```python
from build123d import *

# Parameters (mm, degrees)
ESBO_O1_W                = 140
ESBO_O1_H                = 100
RESSALTO_EXTRUS_O1_DEPTH = 1.5
RESSALTO_EXTRUS_O2_DEPTH = 3
ESBO_O2_R                = 1.5
CORTE_EXTRUS_O1_DEPTH    = 95.451045521
CUT_EXTRUDE1_DEPTH       = 95.451045521
CUT_EXTRUDE1_DEPTH_BACK  = 95.451045521
SKETCH1_R                = 1.7
CUT_EXTRUDE4_DEPTH       = 95.415305963
CUT_EXTRUDE4_DEPTH_BACK  = 95.415305963
FILLET1_R                = 1
CUT_EXTRUDE3_DEPTH       = 95.415305963
CUT_EXTRUDE3_DEPTH_BACK  = 95.415305963
SKETCH2_W                = 3.2
SKETCH2_H                = 15.2


with BuildPart() as part:
    # Esboço1 → Ressalto-extrusão1 (new, symmetric)
    with BuildSketch(Plane(origin=(0, 0, 0), x_dir=(1, 0, 0), z_dir=(0, 1, 0))):
        Rectangle(ESBO_O1_W, ESBO_O1_H)
    extrude(amount=RESSALTO_EXTRUS_O1_DEPTH, both=True)

    # Esboço4 → Ressalto-extrusão2 (add, through all)
    with BuildSketch(Plane(origin=(0, 1.5, 0), x_dir=(1, 0, 0), z_dir=(0, 1, 0))):
        with BuildLine():
            Line((6.5, 53), (20, 53))
            Line((20, 53), (20, 50))
            Line((20, 50), (-20, 50))
            Line((-20, 50), (-20, 53))
            Line((-20, 53), (-6.5, 53))
            ThreePointArc((-6.5, 53), (-5.085786438, 53.585786438), (-4.5, 55))
            Line((-4.5, 55), (-4.5, 56))
            Line((-4.5, 56), (4.5, 56))
            Line((4.5, 56), (4.5, 55))
            ThreePointArc((4.5, 55), (5.085786438, 53.585786438), (6.5, 53))
        make_face()
        with BuildLine():
            Line((4.5, -56), (4.5, -55))
            ThreePointArc((4.5, -55), (5.085786438, -53.585786438), (6.5, -53))
            Line((6.5, -53), (20, -53))
            Line((20, -53), (20, -50))
            Line((20, -50), (-20, -50))
            Line((-20, -50), (-20, -53))
            Line((-20, -53), (-6.5, -53))
            ThreePointArc((-6.5, -53), (-5.085786438, -53.585786438), (-4.5, -55))
            Line((-4.5, -55), (-4.5, -56))
            Line((-4.5, -56), (4.5, -56))
        make_face()
        with BuildLine():
            Line((70, 20), (73, 20))
            Line((73, 20), (73, 6.5))
            ThreePointArc((73, 6.5), (73.585786438, 5.085786438), (75, 4.5))
            Line((75, 4.5), (76, 4.5))
            Line((76, 4.5), (76, -4.5))
            Line((76, -4.5), (75, -4.5))
            ThreePointArc((75, -4.5), (73.585786438, -5.085786438), (73, -6.5))
            Line((73, -6.5), (73, -20))
            Line((73, -20), (70, -20))
            Line((70, -20), (70, 20))
        make_face()
        with BuildLine():
            Line((-70, 39.5), (-73, 39.5))
            Line((-73, 39.5), (-73, 36))
            ThreePointArc((-73, 36), (-73.585786438, 34.585786438), (-75, 34))
            Line((-75, 34), (-76, 34))
            Line((-76, 34), (-76, 25))
            Line((-76, 25), (-75, 25))
            ThreePointArc((-75, 25), (-73.585786438, 24.414213562), (-73, 23))
            Line((-73, 23), (-73, 19.5))
            Line((-73, 19.5), (-70, 19.5))
            Line((-70, 19.5), (-70, 39.5))
        make_face()
        with BuildLine():
            Line((-76, -34), (-76, -25))
            Line((-76, -25), (-75, -25))
            ThreePointArc((-75, -25), (-73.585786438, -24.414213562), (-73, -23))
            Line((-73, -23), (-73, -19.5))
            Line((-73, -19.5), (-70, -19.5))
            Line((-70, -19.5), (-70, -39.5))
            Line((-70, -39.5), (-73, -39.5))
            Line((-73, -39.5), (-73, -36))
            ThreePointArc((-73, -36), (-73.585786438, -34.585786438), (-75, -34))
            Line((-75, -34), (-76, -34))
        make_face()
    extrude(amount=-RESSALTO_EXTRUS_O2_DEPTH)

    # Esboço2 → Corte-extrusão1 (cut, through all)
    with BuildSketch(Plane(origin=(0, 1.5, 0), x_dir=(1, 0, 0), z_dir=(0, 1, 0))):
        with Locations(Location((0, -51.5, 0), (0, 0, 270))):
            Circle(ESBO_O2_R)
        with Locations(Location((0, 51.5, 0), (0, 0, 90))):
            Circle(ESBO_O2_R)
        with Locations(Location((71.5, 0, 0), (0, 0, 90))):
            Circle(ESBO_O2_R)
        with Locations(Location((-71.5, 29.5, 0), (0, 0, 270))):
            Circle(ESBO_O2_R)
        with Locations(Location((-71.5, -29.5, 0), (0, 0, 90))):
            Circle(ESBO_O2_R)
    extrude(amount=-CORTE_EXTRUS_O1_DEPTH, mode=Mode.SUBTRACT)

    # Sketch1 → Cut-Extrude1 (cut, two sides: drawn at the far end of the back side and taken through both)
    with BuildSketch(Plane(origin=(0, 1.5, 0), x_dir=(1, 0, 0), z_dir=(0, 1, 0)).offset(-CUT_EXTRUDE1_DEPTH_BACK)):
        with Locations(Location((30.5, -22.15, 0), (0, 0, 270))):
            Circle(SKETCH1_R)
        with Locations(Location((37.9, -22.15, 0), (0, 0, 270))):
            Circle(SKETCH1_R)
        with Locations(Location((37.9, 22.15, 0), (0, 0, 90))):
            Circle(SKETCH1_R)
        with Locations(Location((30.5, 22.15, 0), (0, 0, 90))):
            Circle(SKETCH1_R)
        with Locations(Location((-30.5, 22.15, 0), (0, 0, 270))):
            Circle(SKETCH1_R)
        with Locations(Location((-37.9, 22.15, 0), (0, 0, 270))):
            Circle(SKETCH1_R)
        with Locations(Location((-37.9, -22.15, 0), (0, 0, 90))):
            Circle(SKETCH1_R)
        with Locations(Location((-30.5, -22.15, 0), (0, 0, 90))):
            Circle(SKETCH1_R)
    extrude(amount=CUT_EXTRUDE1_DEPTH + CUT_EXTRUDE1_DEPTH_BACK, mode=Mode.SUBTRACT)

    # Sketch3 → Cut-Extrude4 (cut, two sides: drawn at the far end of the back side and taken through both)
    with BuildSketch(Plane(origin=(0, 0, 0), x_dir=(1, 0, 0), z_dir=(0, 1, 0)).offset(-CUT_EXTRUDE4_DEPTH_BACK)):
        with BuildLine():
            Line((-70, 3), (-66, 3))
            ThreePointArc((-66, 3), (-65.292893219, 2.707106781), (-65, 2))
            Line((-65, 2), (-65, -2))
            ThreePointArc((-65, -2), (-65.292893219, -2.707106781), (-66, -3))
            Line((-66, -3), (-70, -3))
            Line((-70, -3), (-70, 3))
        make_face()
        with BuildLine():
            Line((-70, 16), (-65.5, 16))
            ThreePointArc((-65.5, 16), (-65.146446609, 15.853553391), (-65, 15.5))
            Line((-65, 15.5), (-65, 13.5))
            ThreePointArc((-65, 13.5), (-65.146446609, 13.146446609), (-65.5, 13))
            Line((-65.5, 13), (-70, 13))
            Line((-70, 13), (-70, 16))
        make_face()
        with BuildLine():
            Line((-65, -15.5), (-65, -13.5))
            ThreePointArc((-65, -13.5), (-65.146446609, -13.146446609), (-65.5, -13))
            Line((-65.5, -13), (-70, -13))
            Line((-70, -13), (-70, -16))
            Line((-70, -16), (-65.5, -16))
            ThreePointArc((-65.5, -16), (-65.146446609, -15.853553391), (-65, -15.5))
        make_face()
    extrude(amount=CUT_EXTRUDE4_DEPTH + CUT_EXTRUDE4_DEPTH_BACK, mode=Mode.SUBTRACT)

    # Fillet1
    fillet1_edges = [part.edges().sort_by_distance(p)[0] for p in [
        (-4.5, 0, -56),
        (4.5, 0, -56),
        (4.5, 0, 56),
        (-4.5, 0, 56),
        (76, 0, 4.5),
        (76, 0, -4.5),
        (-76, 0, 25),
        (-76, 0, 34),
        (-76, 0, -25),
        (-76, 0, -34),
        (-70, 0, 3),
        (-70, 0, -3),
        (-70, 0, -16),
        (-70, 0, -13),
        (-70, 0, 16),
        (-70, 0, 13),
    ]]
    fillet(fillet1_edges, radius=FILLET1_R - 0.0001)  # a hair under: the kernel refuses the full size

    # Sketch2 → Cut-Extrude3 (cut, two sides: drawn at the far end of the back side and taken through both)
    with BuildSketch(Plane(origin=(0, 0, 0), x_dir=(1, 0, 0), z_dir=(0, 1, 0)).offset(-CUT_EXTRUDE3_DEPTH_BACK)):
        with Locations((61.4, 0)):
            Rectangle(SKETCH2_W, SKETCH2_H)
    extrude(amount=CUT_EXTRUDE3_DEPTH + CUT_EXTRUDE3_DEPTH_BACK, mode=Mode.SUBTRACT)


solid = part.part
```
Design review of the part built by this model. Coordinates are the model's own, in mm. A direction names the side the tool comes from. Coordinates: 2 decimals unless noted, no trailing zeros. Order: outer loops, then holes, each group sorted by start corner. A loop starts at its lowest first (then second) coordinate and runs counter-clockwise, first axis right, second up.
1) Mouldability with a two-part tool opening along X and no side actions: class faces 5 (the flat face through (-71, 0, -39.5)), 6 (the flat face through (70, 0, -35)), 7 (the cylindrical face through (31.2, 0, -23.7)) as +X half, -X half, draft (parallel to the pull), parting line (faces both ways), or undercut.
2) Take a section at C-C, the plane z = -47.5. Give the boundary of the cut face in (x, y).
3) Take a section at D-D, the plane x = 55. Give the boundary of the cut face in (y, z).
4) For faces 1 (the flat face through (-73, 0, 21)), 2 (the flat face through (-73, 0, -38)), 3 (the flat face through (45, 0, 50)), 4 (the flat face through (-70, 0, 45)), list the 3-axis set-ups (+Z, -Z, +X, -X, +Y, -Y) from which the entire face can be reached by the end or side of a thin tool; tool diameter is ignored.
5) Take a section at A-A, the plane x = 37.9. Give the boundary of the cut face in (y, z).
6) Clearance check with flat-ended pins moving along their axes: pin 1 (2.5 mm diameter, centred on x = -30.5, z = -22.15, fed in from -Y); pin 2 (1.5 mm diameter, centred on y = -0.5, z = -9.5, fed in from -X); pin 3 (1.5 mm diameter, centred on x = 71.5, y = -0.5, fed in from +Z); pin 4 (1.5 mm diameter, centred on x = 34, y = -0.5, fed in from -Z). State where each tip first meets the part, or that it passes through.
7) Wall thickness on line 1 along X through (y, z) = (-0.7, 22.15); line 2 along X through (y, z) = (0.65, 0); line 3 along X through (y, z) = (-0.7, -51.5): over which ranges is each line inside the solid? List them lowest first.
8) Take a section at B-B, the plane y = -0.1. State how many separate pieces and enclosed holes the cut face has, and give its area (3 significant figures).
Returned:
1. face 5: draft
1. face 6: +X half
1. face 7: undercut
2. outline: (-70, -1.5) - (70, -1.5) - (70, 1.5) - (-70, 1.5) - close
3. outline: (-1.5, -50) - (1.5, -50) - (1.5, 50) - (-1.5, 50) - close
4. face 1: -X, +Y, -Y
4. face 2: -Z, -X, +Y, -Y
4. face 3: +Z, +X, +Y, -Y
4. face 4: +Z, -X, +Y, -Y
5. outline: (-1.5, -50) - (1.5, -50) - (1.5, -23.85) - (-1.5, -23.85) - close; (-1.5, -20.45) - (1.5, -20.45) - (1.5, 20.45) - (-1.5, 20.45) - close; (-1.5, 23.85) - (1.5, 23.85) - (1.5, 50) - (-1.5, 50) - close
6. pin 1: passes through
6. pin 2: stops at x = -70
6. pin 3: stops at z = 20
6. pin 4: stops at z = -50
7. line 1: x = -73 to -39.6, -36.2 to -32.2, -28.8 to 28.8, 32.2 to 36.2, 39.6 to 70
7. line 2: x = -65 to 59.8, 63 to 70, 73 to 76
7. line 3: x = -20 to -1.5, 1.5 to 20
8. separate pieces: 1
8. enclosed holes: 14
8. area: 14,400 mm2
